Verification items for the finished model (mm, model axes). A direction names the side the tool comes from. Round coordinates to 2 decimals unless told otherwise and drop trailing zeros. Use CSV: the item, a comma, the result in double quotes. Start each with the question number.
```python
from build123d import *

# Parameters (mm, degrees)
F1_DEPTH = 3.175
F3_DEPTH = 1.5875
F4_W     = 25.4
F4_H     = 1.27
F5_DEPTH = 25.4
F7_DEPTH = 0.79375


with BuildPart() as f1:
    # F0 (on Top) → F1 (new body)
    with BuildSketch(Plane.XY):
        with BuildLine():
            ThreePointArc((50.8, 38.1), (47.080256, 47.080256), (38.1, 50.8))
            Line((38.1, 50.8), (-38.1, 50.8))
            ThreePointArc((-38.1, 50.8), (-47.080256, 47.080256), (-50.8, 38.1))
            Line((-50.8, 38.1), (-50.8, -38.1))
            ThreePointArc((-50.8, -38.1), (-47.080256, -47.080256), (-38.1, -50.8))
            Line((-38.1, -50.8), (38.1, -50.8))
            ThreePointArc((38.1, -50.8), (47.080256, -47.080256), (50.8, -38.1))
            Line((50.8, -38.1), (50.8, 38.1))
        make_face()
    extrude(amount=F1_DEPTH)

    # F2 (on face) → F3 (cut)
    with BuildSketch(Plane(origin=(0, 0, 0), x_dir=(1, 0, 0), z_dir=(0, 0, -1))):
        with BuildLine():
            ThreePointArc((44.45, 38.1), (42.590128, 42.590128), (38.1, 44.45))
            Line((38.1, 44.45), (-38.1, 44.45))
            ThreePointArc((-38.1, 44.45), (-42.590128, 42.590128), (-44.45, 38.1))
            Line((-44.45, 38.1), (-44.45, -38.1))
            ThreePointArc((-44.45, -38.1), (-42.590128, -42.590128), (-38.1, -44.45))
            Line((-38.1, -44.45), (38.1, -44.45))
            ThreePointArc((38.1, -44.45), (42.590128, -42.590128), (44.45, -38.1))
            Line((44.45, -38.1), (44.45, 38.1))
        make_face()
    extrude(amount=-F3_DEPTH, mode=Mode.SUBTRACT)

    # F4 (on face) → F5 (cut)
    with BuildSketch(Plane.XZ.offset(50.8)):
        with Locations((0, 0.635)):
            Rectangle(F4_W, F4_H)
        with Locations((0, -0.635)):
            Rectangle(F4_W, F4_H)
    extrude(amount=-F5_DEPTH, mode=Mode.SUBTRACT)

    # F6 (on face) → F7 (join)
    with BuildSketch(Plane.XY.offset(3.175)):
        with BuildLine():
            Line((-38.0365, -44.3865), (38.0365, -44.3865))
            ThreePointArc((38.0365, -44.3865), (42.526628, -42.526628), (44.3865, -38.0365))
            Line((44.3865, -38.0365), (44.3865, 38.0365))
            ThreePointArc((44.3865, 38.0365), (42.526628, 42.526628), (38.0365, 44.3865))
            Line((38.0365, 44.3865), (-38.0365, 44.3865))
            ThreePointArc((-38.0365, 44.3865), (-42.526628, 42.526628), (-44.3865, 38.0365))
            Line((-44.3865, 38.0365), (-44.3865, -38.0365))
            ThreePointArc((-44.3865, -38.0365), (-42.526628, -42.526628), (-38.0365, -44.3865))
        make_face()
        with BuildLine():
            ThreePointArc((38.0365, 43.116499), (41.628602, 41.628602), (43.116499, 38.0365))
            Line((43.116499, 38.0365), (43.116499, -38.0365))
            ThreePointArc((43.116499, -38.0365), (41.628602, -41.628602), (38.0365, -43.116499))
            Line((38.0365, -43.116499), (-38.0365, -43.116499))
            ThreePointArc((-38.0365, -43.116499), (-41.628602, -41.628602), (-43.116499, -38.0365))
            Line((-43.116499, -38.0365), (-43.116499, 38.0365))
            ThreePointArc((-43.116499, 38.0365), (-41.628602, 41.628602), (-38.0365, 43.116499))
            Line((-38.0365, 43.116499), (38.0365, 43.116499))
        make_face(mode=Mode.SUBTRACT)
    extrude(amount=F7_DEPTH)


solid = f1.part
```
Q1. Tool access check on faces 4 (the face through (-42.64, 42.54, 0.78)), 5 (the face through (41.668, -41.589, 3.566)), 6 (the face through (42.576, 42.477, 3.566)), 7 (the face through (47.18, 46.98, 1.57)), 8 (the face through (-42.576, -42.477, 3.566)). Record the directions out of +Z, -Z, +X, -X, +Y, -Y that give a thin tool (end or side, any length) a straight path to the whole face; none if there is none.
Q2. Depth check by flat-ended pin: pin 1 Ø1 at (y, z) = (-48.5, 0.5) entering from -X; pin 2 Ø7 at (x, y) = (4, -47) entering from -Z; pin 3 Ø1 at (y, z) = (-49, 1) entering from +X. Enter the tip coordinate at first touch or a pass-through.
Q3. Thickness scan on L1, parallel to Y at x = 19, z = 1.2; L2, parallel to Z at x = -25.5, y = 25 (1 decimal). Record the ranges inside material, lowest first. Write a range as from..to.
Q4. Release check for a two-part mould opening along Y. For faces 1 (the face through (-47.18, -46.98, 1.57)), 2 (the face through (-41.668, 41.589, 3.566)), 3 (the face through (0, 45, 0)) record: +Y half, -Y half, draft (parallel to the pull), parting line (faces both ways), or undercut.
Answer list:
1,face 4,"-Z"
1,face 5,"+Z"
1,face 6,"+Z, +X, +Y"
1,face 7,"+Z, -Z, +X, +Y"
1,face 8,"+Z, -X, -Y"
2,pin 1,"stops at x = -46.05"
2,pin 2,"stops at z = 1.27"
2,pin 3,"stops at x = 45.39"
3,L1,"y = -50.8..-44.45, 44.45..50.8"
3,L2,"z = 1.6..3.2"
4,face 1,"-Y half"
4,face 2,"undercut"
4,face 3,"draft"
